Can you work these out from the drawing? Everything is in mm from the part's minimum corner. A direction names the side the tool comes from. Coordinates: 2 decimals unless noted, no trailing zeros. Loops run counter-clockwise (first coordinate to the right, second up) from the corner with the lowest first, then second, coordinate; pieces in that order, holes last. Notation, with made-up numbers: (-12.75, 87) - (42.25, 87) arc R22 ccw to (42.25, 101) - close; hole circle Ø2 at (-28.75, 62.25). An arc over 180 degrees is marked (long way). Put each result on its own line as item: value. Start each with the question number.
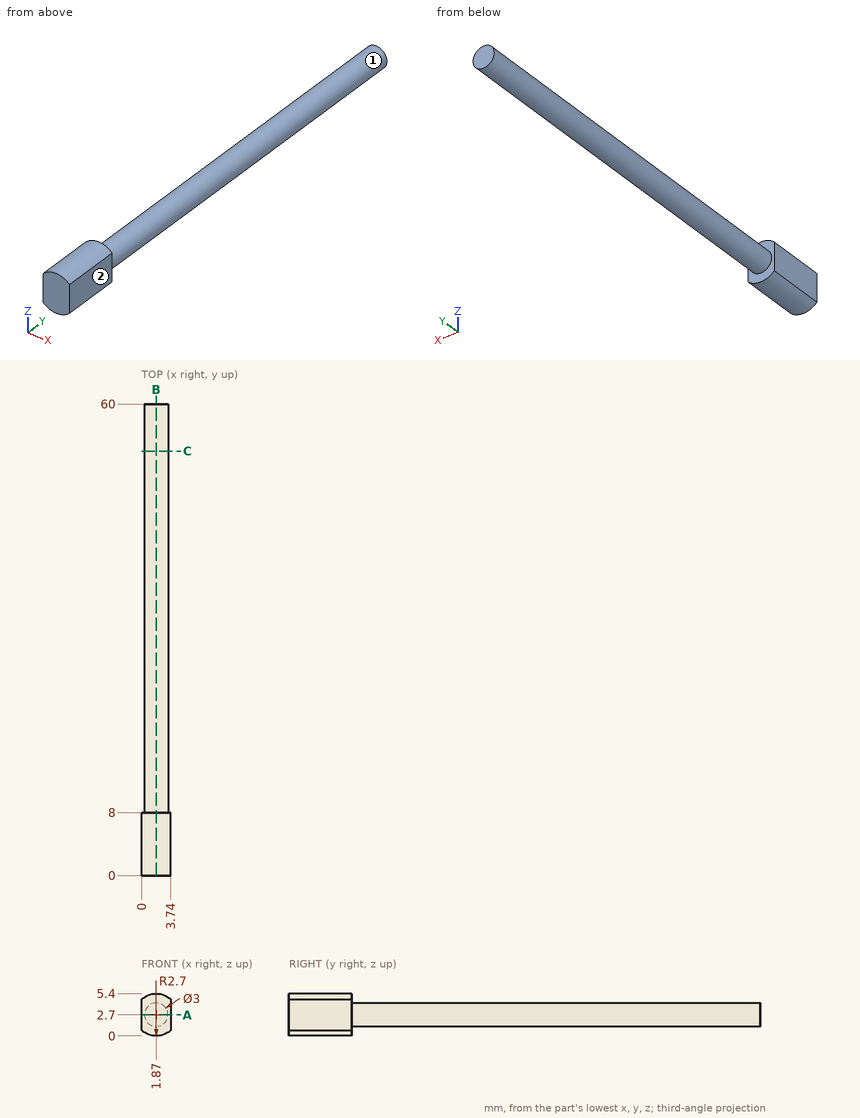
Q1. Will these pins go through, and if not, where does the flat tip stop? pin 1 (1 mm diameter, centred on x = 1, z = 2.5, fed in from -Y); pin 2 (1 mm diameter, centred on y = 52, z = 1.5, fed in from -X).
Q2. Please list where these lines run through material, in increasing order: line 1 along Y through (x, z) = (0.45, 1.1); line 2 along Z through (x, y) = (2, 29); line 3 along X through (y, z) = (18.5, 3.85). Write a range as [from, to].
Q3. I want a section at A-A on z = 2.7. List the corners of the cut face in (x, y) for me, and give its area (3 significant figures).
Q4. On a 3-axis mill with a long thin cutter (end or side, diameter ignored), from which of +Z, -Z, +X, -X, +Y, -Y can I reach the whole of each face in a straight line? I mean the marked faces 1 and 2. Say none if no direction works.
Q5. I want a section at B-B on x = 1.87. List the corners of the cut face in (y, z) for me.
Q6. I want a section at C-C on y = 54. List the corners of the cut face in (x, z) for me, and give its area (3 significant figures).
Calculated:
1. pin 1: y = 0
1. pin 2: x = 0.54
2. line 1: [0, 8]
2. line 2: [1.21, 4.19]
2. line 3: [0.91, 2.83]
3. outline: (0, 0) - (3.74, 0) - (3.74, 8) - (3.37, 8) - (3.37, 60) - (0.37, 60) - (0.37, 8) - (0, 8) - close
3. area: 186 mm2
4. face 1: +Y
4. face 2: +Z, -Z, +X, +Y, -Y
5. outline: (0, 0) - (8, 0) - (8, 1.2) - (60, 1.2) - (60, 4.2) - (8, 4.2) - (8, 5.4) - (0, 5.4) - close
6. outline: circle Ø3 at (1.87, 2.7)
6. area: 7.07 mm2
